from build123d import *

# Parameters (mm, degrees)
SKETCH1_R           = 3
SKETCH1_R_2         = 2.25
SKETCH1_R_3         = 1.75
SKETCH1_R_4         = 14.5
SKETCH1_R_5         = 1.77
SKETCH1_R_6         = 1.8
SKETCH1_R_7         = 5
BOSS_EXTRUDE1_DEPTH = 5


with BuildPart() as part:
    # Sketch1 → Boss-Extrude1 (new body)
    with BuildSketch(Plane.XY):
        with BuildLine():
            Line((119, 137.85), (-117, 137.85))
            ThreePointArc((-117, 137.85), (-118.414213562, 137.264213563), (-119, 135.85))
            Line((-119, 135.85), (-119, 131.85))
            ThreePointArc((-119, 131.85), (-119.585786438, 130.435786438), (-121, 129.85))
            Line((-121, 129.85), (-141, 129.85))
            ThreePointArc((-141, 129.85), (-142.414213562, 129.264213563), (-143, 127.85))
            Line((-143, 127.85), (-143, -101.5))
            ThreePointArc((-143, -101.5), (-142.853553391, -101.853553391), (-142.5, -102))
            Line((-142.5, -102), (-128.5, -102))
            ThreePointArc((-128.5, -102), (-128.14644661, -102.146446609), (-128, -102.5))
            Line((-128, -102.5), (-128, -126.5))
            ThreePointArc((-128, -126.5), (-128.14644661, -126.853553391), (-128.5, -127))
            Line((-128.5, -127), (-142.5, -127))
            ThreePointArc((-142.5, -127), (-142.853553391, -127.146446609), (-143, -127.5))
            Line((-143, -127.5), (-143, -147))
            ThreePointArc((-143, -147), (-142.121320344, -149.121320344), (-140, -150))
            Line((-140, -150), (142, -150))
            ThreePointArc((142, -150), (144.121320344, -149.121320344), (145, -147))
            Line((145, -147), (145, 127.85))
            ThreePointArc((145, 127.85), (144.414213562, 129.264213563), (143, 129.85))
            Line((143, 129.85), (123, 129.85))
            ThreePointArc((123, 129.85), (121.585786438, 130.435786438), (121, 131.85))
            Line((121, 131.85), (121, 135.85))
            ThreePointArc((121, 135.85), (120.414213562, 137.264213563), (119, 137.85))
        make_face()
        with Locations((132, -137)):
            Circle(SKETCH1_R, mode=Mode.SUBTRACT)
        with Locations((-130, -136.98801067)):
            Circle(SKETCH1_R, mode=Mode.SUBTRACT)
        with Locations((80.1, 120.55)):
            Circle(SKETCH1_R_2, mode=Mode.SUBTRACT)
        with Locations((101.9, 124.85)):
            Circle(SKETCH1_R_2, mode=Mode.SUBTRACT)
        with Locations((100.1, 112.65)):
            Circle(SKETCH1_R_2, mode=Mode.SUBTRACT)
        with Locations((-85.403167437, 119.6)):
            Circle(SKETCH1_R_2, mode=Mode.SUBTRACT)
        with Locations((-105.303167437, 112)):
            Circle(SKETCH1_R_2, mode=Mode.SUBTRACT)
        with Locations((-106.903167437, 123.8)):
            Circle(SKETCH1_R_2, mode=Mode.SUBTRACT)
        with Locations((-84.791108936, -35.5)):
            Circle(SKETCH1_R_3, mode=Mode.SUBTRACT)
        with Locations((45.999972222, -0.949999618)):
            Circle(SKETCH1_R_2, mode=Mode.SUBTRACT)
        with Locations((-84.791108936, -65.5)):
            Circle(SKETCH1_R_3, mode=Mode.SUBTRACT)
        with Locations((-43.999972222, -1.050000381)):
            Circle(SKETCH1_R_2, mode=Mode.SUBTRACT)
        with Locations((72.5, 79.5)):
            Circle(SKETCH1_R_4, mode=Mode.SUBTRACT)
        with Locations((-31.791108936, -65.5)):
            Circle(SKETCH1_R_3, mode=Mode.SUBTRACT)
        with Locations((72.5, 60)):
            Circle(SKETCH1_R_3, mode=Mode.SUBTRACT)
        with Locations((72.5, 99)):
            Circle(SKETCH1_R_3, mode=Mode.SUBTRACT)
        with Locations((-10.373326807, -65.5)):
            Circle(SKETCH1_R_3, mode=Mode.SUBTRACT)
        with Locations((42.626673193, -65.5)):
            Circle(SKETCH1_R_3, mode=Mode.SUBTRACT)
        with Locations((42.626673193, -35.5)):
            Circle(SKETCH1_R_3, mode=Mode.SUBTRACT)
        with Locations((-31.791108936, -35.5)):
            Circle(SKETCH1_R_3, mode=Mode.SUBTRACT)
        with Locations((-10.373326807, -35.5)):
            Circle(SKETCH1_R_3, mode=Mode.SUBTRACT)
        with Locations((-33, 27.5)):
            Circle(SKETCH1_R_3, mode=Mode.SUBTRACT)
        with Locations((-33, -2)):
            Circle(SKETCH1_R_3, mode=Mode.SUBTRACT)
        with Locations((12, 27.5)):
            Circle(SKETCH1_R_3, mode=Mode.SUBTRACT)
        with Locations((12, -2)):
            Circle(SKETCH1_R_3, mode=Mode.SUBTRACT)
        with Locations((12.5, 113.5)):
            Circle(SKETCH1_R_3, mode=Mode.SUBTRACT)
        with Locations((12.5, 102.46)):
            Circle(SKETCH1_R_3, mode=Mode.SUBTRACT)
        with Locations((32.5, 113.5)):
            Circle(SKETCH1_R_3, mode=Mode.SUBTRACT)
        with Locations((32.5, 102.46)):
            Circle(SKETCH1_R_3, mode=Mode.SUBTRACT)
        with Locations((12.5, 53.54)):
            Circle(SKETCH1_R_3, mode=Mode.SUBTRACT)
        with Locations((32.5, 53.54)):
            Circle(SKETCH1_R_3, mode=Mode.SUBTRACT)
        with Locations((32.5, 42.5)):
            Circle(SKETCH1_R_5, mode=Mode.SUBTRACT)
        with Locations((12.5, 42.5)):
            Circle(SKETCH1_R_3, mode=Mode.SUBTRACT)
        with Locations((45.752852724, 22.5)):
            Circle(SKETCH1_R_3, mode=Mode.SUBTRACT)
        with Locations((56.792852724, 22.5)):
            Circle(SKETCH1_R_3, mode=Mode.SUBTRACT)
        with Locations((61.46, -17.5)):
            Circle(SKETCH1_R_3, mode=Mode.SUBTRACT)
        with Locations((72.5, -17.5)):
            Circle(SKETCH1_R_3, mode=Mode.SUBTRACT)
        with Locations((-80.5, 23.5)):
            Circle(SKETCH1_R_3, mode=Mode.SUBTRACT)
        with Locations((-80.5, 12.46)):
            Circle(SKETCH1_R_3, mode=Mode.SUBTRACT)
        with Locations((112.5, 93.54)):
            Circle(SKETCH1_R_3, mode=Mode.SUBTRACT)
        with Locations((112.5, 82.5)):
            Circle(SKETCH1_R_3, mode=Mode.SUBTRACT)
        with Locations((107.5, 63.5)):
            Circle(SKETCH1_R_3, mode=Mode.SUBTRACT)
        with Locations((107.5, 52.46)):
            Circle(SKETCH1_R_3, mode=Mode.SUBTRACT)
        with Locations((-80.5, 73.5)):
            Circle(SKETCH1_R_3, mode=Mode.SUBTRACT)
        with Locations((-80.5, 62.46)):
            Circle(SKETCH1_R_6, mode=Mode.SUBTRACT)
        with Locations((87.25, -132.25)):
            Circle(SKETCH1_R_7, mode=Mode.SUBTRACT)
        with Locations((77.25, -132.25)):
            Circle(SKETCH1_R_3, mode=Mode.SUBTRACT)
        with Locations((97.25, -132.25)):
            Circle(SKETCH1_R_3, mode=Mode.SUBTRACT)
        with BuildLine():
            Line((7.701292612, -14.765451744), (19.701292612, -14.765451744))
            ThreePointArc((19.701292612, -14.765451744), (29.701292612, -24.765451744), (19.701292612, -34.765451744))
            Line((19.701292612, -34.765451744), (7.701292612, -34.765451744))
            ThreePointArc((7.701292612, -34.765451744), (-2.298707388, -24.765451744), (7.701292612, -14.765451744))
        make_face(mode=Mode.SUBTRACT)
        with BuildLine():
            Line((-89.211061563, -78.889424509), (-44.211061563, -79.423092657))
            ThreePointArc((-44.211061563, -79.423092657), (-36.800527355, -87.01150374), (-44.388938437, -94.422037947))
            Line((-44.388938437, -94.422037947), (-89.388938437, -93.888369799))
            ThreePointArc((-89.388938437, -93.888369799), (-96.799472645, -86.299958717), (-89.211061563, -78.889424509))
        make_face(mode=Mode.SUBTRACT)
        with BuildLine():
            Line((-20.765442271, 82.042263173), (-21.760088994, 88.603452442))
            add(Edge.make_bspline(
                [(-21.760088994, 88.603452442), (-15.581917564, 92.98846813), (-11.286155824, 98.883660406), (-8.99377257, 106.126506389)],
                knots=[0, 0, 0, 0, 0.918480676, 0.918480676, 0.918480676, 0.918480676], degree=3))
            ThreePointArc((-8.99377257, 106.126506389), (-8.165849028, 106.816854641), (-7.192132058, 106.35434695))
            add(Edge.make_bspline(
                [(-7.192132058, 106.35434695), (-5.951098608, 104.366564333), (-4.534413043, 100.165736474), (-4.849455476, 88.003219654), (-9.488562584, 76.016189543), (-20.765442271, 82.042263173)],
                knots=[0.050637749, 0.050637749, 0.050637749, 0.050637749, 0.222928156, 0.39163585, 1, 1, 1, 1], degree=3))
        make_face(mode=Mode.SUBTRACT)
        with BuildLine():
            Line((-30.72614089, 78.073067173), (-24.164951621, 79.067713897))
            add(Edge.make_bspline(
                [(-24.164951621, 79.067713897), (-19.779935933, 72.889542467), (-13.884743657, 68.593780727), (-6.641897674, 66.301397473)],
                knots=[0, 0, 0, 0, 0.918480676, 0.918480676, 0.918480676, 0.918480676], degree=3))
            ThreePointArc((-6.641897674, 66.301397473), (-5.951549422, 65.47347393), (-6.414057113, 64.49975696))
            add(Edge.make_bspline(
                [(-6.414057113, 64.49975696), (-8.40183973, 63.25872351), (-12.602667589, 61.842037945), (-24.765184409, 62.157080378), (-36.75221452, 66.796187486), (-30.72614089, 78.073067173)],
                knots=[0.050637749, 0.050637749, 0.050637749, 0.050637749, 0.222928156, 0.39163585, 1, 1, 1, 1], degree=3))
        make_face(mode=Mode.SUBTRACT)
        with BuildLine():
            Line((-34.69533689, 88.033765792), (-33.700690166, 81.472576523))
            add(Edge.make_bspline(
                [(-33.700690166, 81.472576523), (-39.878861596, 77.087560835), (-44.174623336, 71.192368559), (-46.46700659, 63.949522577)],
                knots=[0, 0, 0, 0, 0.918480676, 0.918480676, 0.918480676, 0.918480676], degree=3))
            ThreePointArc((-46.46700659, 63.949522577), (-47.294930133, 63.259174324), (-48.268647103, 63.721682015))
            add(Edge.make_bspline(
                [(-48.268647103, 63.721682015), (-49.509680553, 65.709464633), (-50.926366118, 69.910292491), (-50.611323685, 82.072809312), (-45.972216577, 94.059839422), (-34.69533689, 88.033765792)],
                knots=[0.050637749, 0.050637749, 0.050637749, 0.050637749, 0.222928156, 0.39163585, 1, 1, 1, 1], degree=3))
        make_face(mode=Mode.SUBTRACT)
        with BuildLine():
            Line((-24.734638271, 92.002961792), (-31.29582754, 91.008315069))
            add(Edge.make_bspline(
                [(-31.29582754, 91.008315069), (-35.680843228, 97.186486499), (-41.576035504, 101.482248239), (-48.818881486, 103.774631493)],
                knots=[0, 0, 0, 0, 0.918480676, 0.918480676, 0.918480676, 0.918480676], degree=3))
            ThreePointArc((-48.818881486, 103.774631493), (-49.509229739, 104.602555035), (-49.046722048, 105.576272005))
            add(Edge.make_bspline(
                [(-49.046722048, 105.576272005), (-47.05893943, 106.817305455), (-42.858111572, 108.23399102), (-30.695594751, 107.918948587), (-18.708564641, 103.279841479), (-24.734638271, 92.002961792)],
                knots=[0.050637749, 0.050637749, 0.050637749, 0.050637749, 0.222928156, 0.39163585, 1, 1, 1, 1], degree=3))
        make_face(mode=Mode.SUBTRACT)
    extrude(amount=BOSS_EXTRUDE1_DEPTH)


solid = part.part
Here's how the part is built. I have some questions about the finished solid (model axes, mm). A direction names the side the tool comes from. Coordinates: 2 decimals unless noted, no trailing zeros. Write each loop counter-clockwise with the first axis right and the second up, starting at its lowest first coordinate (ties: lowest second). Pieces come first, ordered by that corner, then holes.
Item 1: If we mould it in two halves opening along Y, with no side actions, what happens to faces 1 (the cylindrical face through (-96.8, -86.5, 2.5)), 2 (the flat face through (-1, -4, 0))? For each: +Y half, -Y half, draft (parallel to the pull), parting line (faces both ways), or undercut.
Item 2: I want a section at A-A on y = -84.5. Write out the boundary of the cut face in (x, z), and give its area (3 significant figures).
Item 3: On a 3-axis mill with a long thin cutter (end or side, diameter ignored), from which of +Z, -Z, +X, -X, +Y, -Y can I reach the whole of each face in a straight line? I mean faces 3 (the cylindrical face through (29.7, -24.55, 2.46)), 4 (the flat face through (-1, -4, 5)). Say none if no direction works.
Item 4: I want a section at C-C on z = 2.95. Count the separate pieces of the cut face and the enclosed holes in it, and give its area (3 significant figures).
Item 5: I want a section at B-B on x = -61.5. Write out the boundary of the cut face in (y, z).
Item 6: Will these pins go through, and if not, where does the flat tip stop? pin 1 (3 mm diameter, centred on y = 134.5, z = 2, fed in from +X); pin 2 (1.5 mm diameter, centred on x = -132, z = 3.5, fed in from +Y).
Item 7: If I drill on line 1 (X direction, y = 120, z = 3.6); line 2 (Y direction, x = 112.5, z = 1.55); line 3 (X direction, y = 23, z = 2.2), over which ranges is the centre line in solid material (lowest first)?
Findings below:
1. face 1: undercut
1. face 2: draft
2. outline: (-143, 0) - (-96.56, 0) - (-96.56, 5) - (-143, 5) - close; (-37.2, 0) - (145, 0) - (145, 5) - (-37.2, 5) - close
2. area: 1,140 mm2
3. face 3: +Z, -Z
3. face 4: +Z, +X, -X, +Y, -Y
4. separate pieces: 1
4. enclosed holes: 54
4. area: 78,400 mm2
5. outline: (-150, 0) - (-94.22, 0) - (-94.22, 5) - (-150, 5) - close; (-79.22, 0) - (137.85, 0) - (137.85, 5) - (-79.22, 5) - close
6. pin 1: stops at x = 121
6. pin 2: stops at y = 129.85
7. line 1: x = -143 to -87.62, -83.19 to 77.92, 82.28 to 145
7. line 2: y = -150 to 80.75, 84.25 to 91.79, 95.29 to 137.85
7. line 3: x = -143 to -82.18, -78.82 to 44.08, 47.43 to 55.12, 58.47 to 145
